Model file for the job. Use its own axes, mm. A direction names the side the tool comes from. Give positions to 0.01 mm unless a question says otherwise; leave off trailing zeros. Write each loop counter-clockwise with the first axis right and the second up, starting at its lowest first coordinate (ties: lowest second). Pieces come first, ordered by that corner, then holes. Notation, with made-up numbers: (16.25, -21.5) - (28.25, -21.5) arc R17 ccw to (28.25, 3.5) - close; hole circle Ø2 at (47.25, 67). An arc over 180 degrees is marked (long way). Use CSV: the item, a comma, the result in double quotes.
from build123d import *

# Parameters (mm, degrees)
BOSS_EXTRUDE1_DEPTH = 3


with BuildPart() as part:
    # Sketch3 → Boss-Extrude1 (new body)
    with BuildSketch(Plane(origin=(0, 0, 0), x_dir=(1, 0, 0), z_dir=(0, 1, 0))):
        with BuildLine():
            Line((0.591679445, -30.420098318), (0.591679445, -37.330098318))
            ThreePointArc((0.591679445, -37.330098318), (-0.908320555, -38.830098318), (-2.408320555, -37.330098318))
            Line((-2.408320555, -37.330098318), (-2.408320555, -30.420098318))
            Line((-2.408320555, -30.420098318), (-8.258320555, -30.420098318))
            Line((-8.258320555, -30.420098318), (-8.258320555, -36.830098318))
            ThreePointArc((-8.258320555, -36.830098318), (-9.758320555, -38.330098318), (-11.258320555, -36.830098318))
            Line((-11.258320555, -36.830098318), (-11.258320555, -30.420098318))
            ThreePointArc((-11.258320555, -30.420098318), (-14.157587017, -30.629396859), (-17.034731178, -31.04363517))
            Line((-17.034731178, -31.04363517), (-15.66681067, -37.305974468))
            ThreePointArc((-15.66681067, -37.305974468), (-16.812150481, -39.091526685), (-18.597702697, -37.946186875))
            Line((-18.597702697, -37.946186875), (-19.965623205, -31.683847576))
            ThreePointArc((-19.965623205, -31.683847576), (-22.753437017, -32.507040171), (-25.475903143, -33.525730554))
            Line((-25.475903143, -33.525730554), (-22.803084936, -39.351890767))
            ThreePointArc((-22.803084936, -39.351890767), (-23.540996482, -41.340731271), (-25.529836986, -40.602819725))
            Line((-25.529836986, -40.602819725), (-28.202655193, -34.776659512))
            ThreePointArc((-28.202655193, -34.776659512), (-30.750576247, -36.175820045), (-33.192934927, -37.752029415))
            Line((-33.192934927, -37.752029415), (-29.338361053, -42.873587796))
            ThreePointArc((-29.338361053, -42.873587796), (-29.634847287, -44.974086764), (-31.735346255, -44.67760053))
            Line((-31.735346255, -44.67760053), (-35.589920129, -39.556042149))
            ThreePointArc((-35.589920129, -39.556042149), (-37.780560653, -41.466708522), (-39.830287583, -43.52781779))
            Line((-39.830287583, -43.52781779), (-34.9715459, -47.708813994))
            ThreePointArc((-34.9715459, -47.708813994), (-34.812947114, -49.824197275), (-36.928330395, -49.982796061))
            Line((-36.928330395, -49.982796061), (-41.787072078, -45.801799857))
            ThreePointArc((-41.787072078, -45.801799857), (-43.519504922, -48.135943884), (-45.082165119, -50.586993661))
            Line((-45.082165119, -50.586993661), (-39.443107485, -53.634800906))
            ThreePointArc((-39.443107485, -53.634800906), (-38.836730639, -55.6676086), (-40.869538333, -56.273985446))
            Line((-40.869538333, -56.273985446), (-46.508595967, -53.226178201))
            ThreePointArc((-46.508595967, -53.226178201), (-47.665748765, -55.785413628), (-48.644932096, -58.417881781))
            Line((-48.644932096, -58.417881781), (-42.547032105, -60.378526572))
            ThreePointArc((-42.547032105, -60.378526572), (-41.520814182, -62.235103199), (-43.37739081, -63.261321122))
            Line((-43.37739081, -63.261321122), (-49.536961833, -61.487121356))
            ThreePointArc((-49.536961833, -61.487121356), (-50.138317317, -64.33104883), (-50.536616569, -67.210442795))
            Line((-50.536616569, -67.210442795), (-44.140315801, -67.629294183))
            ThreePointArc((-44.140315801, -67.629294183), (-42.741536695, -69.22410358), (-44.336346092, -70.622882686))
            Line((-44.336346092, -70.622882686), (-50.73264686, -70.204031298))
            ThreePointArc((-50.73264686, -70.204031298), (-50.713243641, -73.110777832), (-50.487893094, -76.008840811))
            Line((-50.487893094, -76.008840811), (-44.149552834, -75.053046508))
            ThreePointArc((-44.149552834, -75.053046508), (-42.442657071, -76.312612644), (-43.702223207, -78.019508408))
            Line((-43.702223207, -78.019508408), (-50.040563467, -78.975302711))
            Line((-50.040563467, -78.975302711), (-48.242175426, -84.448330276))
            Line((-48.242175426, -84.448330276), (-41.903835167, -83.492535972))
            ThreePointArc((-41.903835167, -83.492535972), (-40.196939403, -84.752102109), (-41.456505539, -86.458997873))
            Line((-41.456505539, -86.458997873), (-47.292325887, -87.339014346))
            Line((-47.292325887, -87.339014346), (-44.496146078, -95.848648873))
            Line((-44.496146078, -95.848648873), (-38.157805818, -94.89285457))
            ThreePointArc((-38.157805818, -94.89285457), (-36.450910055, -96.152420706), (-37.710476191, -97.85931647))
            Line((-37.710476191, -97.85931647), (-43.546296539, -98.739332944))
            Line((-43.546296539, -98.739332944), (-40.75011673, -107.248967471))
            Line((-40.75011673, -107.248967471), (-34.41177647, -106.293173167))
            ThreePointArc((-34.41177647, -106.293173167), (-32.704880706, -107.552739304), (-33.964446843, -109.259635067))
            Line((-33.964446843, -109.259635067), (-39.800267191, -110.139651541))
            Line((-39.800267191, -110.139651541), (-37.004087382, -118.649286068))
            Line((-37.004087382, -118.649286068), (-30.665747122, -117.693491765))
            ThreePointArc((-30.665747122, -117.693491765), (-28.958851358, -118.953057901), (-30.218417495, -120.659953665))
            Line((-30.218417495, -120.659953665), (-36.054237843, -121.539970138))
            Line((-36.054237843, -121.539970138), (-35.590669818, -122.95075011))
            ThreePointArc((-35.590669818, -122.95075011), (-34.806974696, -125.75946708), (-34.281042725, -128.627648207))
            Line((-34.281042725, -128.627648207), (-27.747875517, -129.78272529))
            ThreePointArc((-27.747875517, -129.78272529), (-26.531936776, -131.520969513), (-28.270180998, -132.736908254))
            Line((-28.270180998, -132.736908254), (-34.00913019, -131.722250511))
            ThreePointArc((-34.00913019, -131.722250511), (-34.075192309, -135.400732769), (-34.561150831, -139.04757253))
            Line((-34.561150831, -139.04757253), (-28.838758854, -142.17116811))
            ThreePointArc((-28.838758854, -142.17116811), (-28.240821524, -144.206474217), (-30.276127631, -144.804411546))
            Line((-30.276127631, -144.804411546), (-35.2935191, -142.065643934))
            ThreePointArc((-35.2935191, -142.065643934), (-36.539745877, -145.545336545), (-38.177184694, -148.858965366))
            Line((-38.177184694, -148.858965366), (-33.824418851, -153.564444036))
            ThreePointArc((-33.824418851, -153.564444036), (-33.906956954, -155.68415804), (-36.026670958, -155.601619937))
            Line((-36.026670958, -155.601619937), (-39.838521376, -151.480888091))
            ThreePointArc((-39.838521376, -151.480888091), (-42.144817333, -154.387016255), (-44.770614017, -157.008041575))
            Line((-44.770614017, -157.008041575), (-42.183941003, -162.772154464))
            ThreePointArc((-42.183941003, -162.772154464), (-42.938330746, -164.754803226), (-44.920979509, -164.000413483))
            Line((-44.920979509, -164.000413483), (-47.185290179, -158.954649194))
            ThreePointArc((-47.185290179, -158.954649194), (-50.311989567, -160.96907207), (-53.650455908, -162.608825429))
            Line((-53.650455908, -162.608825429), (-53.043901057, -168.832254262))
            ThreePointArc((-53.043901057, -168.832254262), (-54.391321871, -170.470685569), (-56.029753178, -169.123264755))
            Line((-56.029753178, -169.123264755), (-56.560978983, -163.672733804))
            ThreePointArc((-56.560978983, -163.672733804), (-57.462718747, -163.939470451), (-58.371875015, -164.179715994))
            Line((-58.371875015, -164.179715994), (-75.571875015, -164.179715994))
            Line((-75.571875015, -164.179715994), (-75.571875015, -178.729715994))
            Line((-75.571875015, -178.729715994), (-61.216696476, -178.729715994))
            ThreePointArc((-61.216696476, -178.729715994), (-59.722431212, -180.360755387), (-61.477773293, -181.706820898))
            Line((-61.477773293, -181.706820898), (-75.571875015, -181.706820898))
            Line((-75.571875015, -181.706820898), (-75.571875015, -188.366820898))
            Line((-75.571875015, -188.366820898), (-69.758711754, -188.366820898))
            ThreePointArc((-69.758711754, -188.366820898), (-59.859029923, -190.690063204), (-51.226648029, -185.315759714))
            ThreePointArc((-51.226648029, -185.315759714), (-46.206239367, -185.643710412), (-42.424378195, -182.325641566))
            ThreePointArc((-42.424378195, -182.325641566), (-37.700409933, -181.777039638), (-34.747980084, -178.048769502))
            ThreePointArc((-34.747980084, -178.048769502), (-29.512633217, -176.679893654), (-26.778625341, -172.010002988))
            ThreePointArc((-26.778625341, -172.010002988), (-21.874415441, -168.945099351), (-20.57382951, -163.310085129))
            ThreePointArc((-20.57382951, -163.310085129), (-16.135510008, -158.759996314), (-17.712581879, -152.602494179))
            ThreePointArc((-17.712581879, -152.602494179), (-12.736952388, -148.661636396), (-14.20790203, -142.487208808))
            ThreePointArc((-14.20790203, -142.487208808), (-11.660768143, -136.316062867), (-15.601751117, -130.927223803))
            ThreePointArc((-15.601751117, -130.927223803), (-13.478300165, -123.764089753), (-19.712761754, -119.646927859))
            ThreePointArc((-19.712761754, -119.646927859), (-18.260622737, -110.862232301), (-25.024542476, -105.071811459))
            ThreePointArc((-25.024542476, -105.071811459), (-23.152070063, -96.871086954), (-28.913917519, -90.742534985))
            ThreePointArc((-28.913917519, -90.742534985), (-27.85022737, -82.916745733), (-32.6317535, -76.630934567))
            ThreePointArc((-32.6317535, -76.630934567), (-31.035937746, -72.094286151), (-32.956658516, -67.685359014))
            ThreePointArc((-32.956658516, -67.685359014), (-28.901785775, -62.503538673), (-29.698658066, -55.972210359))
            ThreePointArc((-29.698658066, -55.972210359), (-22.933977183, -54.354119985), (-19.255807876, -48.450714658))
            ThreePointArc((-19.255807876, -48.450714658), (-13.273954555, -50.167914793), (-7.839177287, -47.135664555))
            ThreePointArc((-7.839177287, -47.135664555), (-3.40315163, -48.973344156), (0.591679445, -46.309378199))
            Line((0.591679445, -46.309378199), (12.675221537, -48.606938304))
            ThreePointArc((12.675221537, -48.606938304), (19.637576869, -47.715252301), (24.735359205, -42.890098318))
            ThreePointArc((24.735359205, -42.890098318), (25.355154173, -42.278520936), (26.210254983, -42.114279345))
            Line((26.210254983, -42.114279345), (33.591679445, -42.890098318))
            Line((33.591679445, -42.890098318), (33.591679445, -28.420098318))
            Line((33.591679445, -28.420098318), (20.741679445, -28.420098318))
            ThreePointArc((20.741679445, -28.420098318), (19.241679445, -26.920098318), (20.741679445, -25.420098318))
            Line((20.741679445, -25.420098318), (33.591679445, -25.420098318))
            Line((33.591679445, -25.420098318), (33.591679445, -22.706623157))
            ThreePointArc((33.591679445, -22.706623157), (32.712999789, -20.585302814), (30.591679445, -19.706623157))
            ThreePointArc((30.591679445, -19.706623157), (14.663884949, -22.465339604), (0.591679445, -30.420098318))
        make_face()
    extrude(amount=BOSS_EXTRUDE1_DEPTH)


solid = part.part
(1) Saw through at B-B, the plane z = 102. List the corners of the cut face in (x, y), then the cut area to 3 significant figures.
Checked values:
outline,"(-42.47, 0) - (-23.28, 0) - (-23.28, 3) - (-42.47, 3) - close"
area,"57.6 mm^2"
(2) Wall check: probe 1 along X at (y, z) = (0.65, 37); probe 2 along Z at (x, y) = (8, 0.45); probe 3 along Z at (x, y) = (-61.5, 2). Give the ranges that are in metal, low to high. Write a range as [from, to].
Checked values:
probe 1,"x = [-32.07, -27.18], [-23.88, -18.8], [-15.73, -11.25], [-8.27, -2.41], [0.59, 33.59]"
probe 2,"z = [25.44, 47.72]"
probe 3,"z = [164.18, 178.73], [181.71, 190.86]"
(3) Saw through at A-A, the plane x = -64.5. List the corners of the cut face in (y, z).
Checked values:
outline,"(0, 164.18) - (3, 164.18) - (3, 178.73) - (0, 178.73) - close; (0, 181.71) - (3, 181.71) - (3, 190.63) - (0, 190.63) - close"
(4) Pull direction Z, two halves, no side cores. Call faces 4 (the face through (-28.928, 1.479, 62.594)), 5 (the face through (-25.3, 0, 104.9)), 6 (the face through (-60.003, 1.479, 190.713)): released by +Z, released by -Z, zero draft, split by the parting line, or undercut.
Checked values:
face 4,"undercut"
face 5,"zero draft"
face 6,"released by +Z"
(5) 3-axis set-ups, long thin cutter, end or side, ignore diameter. For faces 1 (the face through (-42.11, 1.48, 154.35)), 2 (the face through (-43.6, 1.5, 54.8)), 3 (the face through (-46.275, 1.479, 185.667)): which of +Z, -Z, +X, -X, +Y, -Y reach the whole face in a straight line?
Checked values:
face 1,"-X, +Y, -Y"
face 2,"+Y, -Y"
face 3,"+Z, +Y, -Y"
(6) Flat gauge pins, fed straight in: P1, Ø12, axis at x = -58.5, z = 71, coming from the +Y side; P2, Ø1.5, axis at x = 10, y = 1, coming from the +Z side; P3, Ø1.5, axis at x = -41, y = 2, coming from the -Z side; P4, Ø0.9, axis at x = 26, y = 2, coming from the +Z side. Where does each tip first touch, or does it go through?
Checked values:
P1,"passes through"
P2,"stops at z = 48.24"
P3,"stops at z = 45.83"
P4,"stops at z = 42.19"
(7) Saw through at C-C, the plane z = 81. List the corners of the cut face in (x, y).
Checked values:
outline,"(-49.38, 0) - (-28.56, 0) - (-28.56, 3) - (-49.38, 3) - close"
